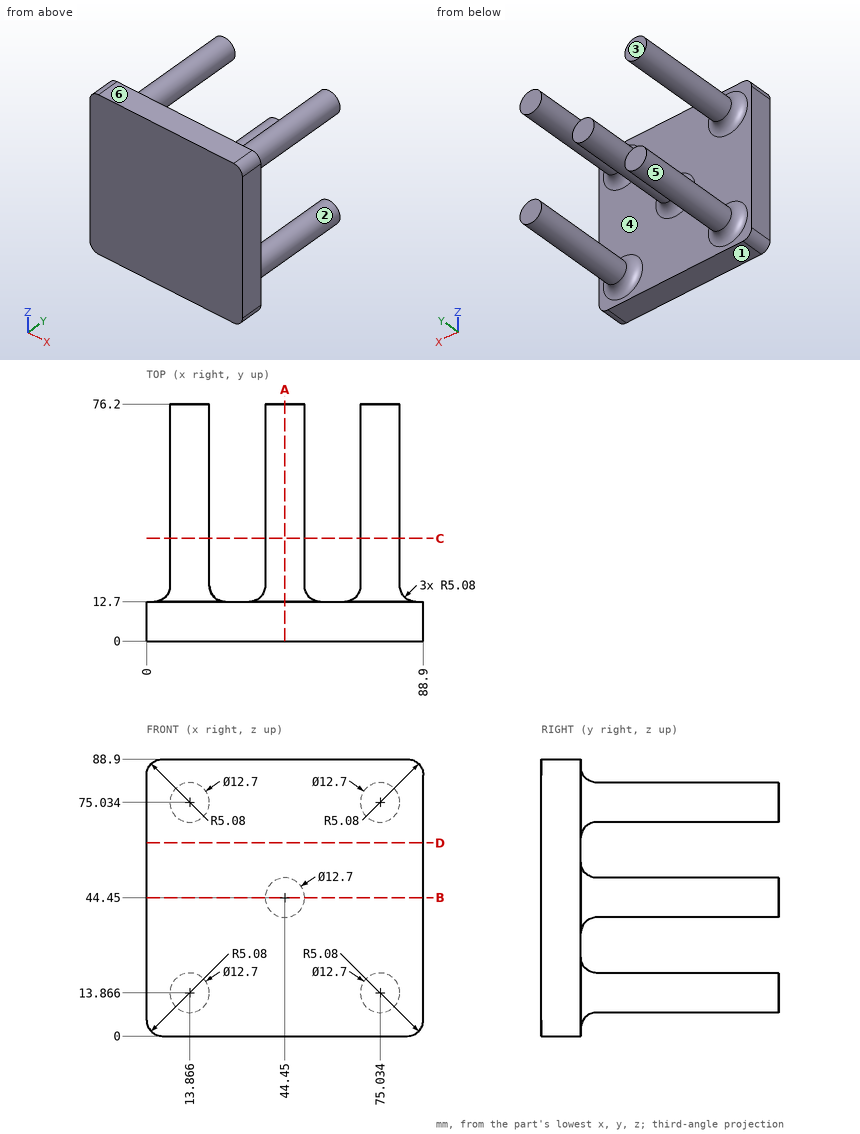
Could you check a few things on this drawing? It's one solid part, dimensions in mm from its lowest x, y, z. A direction names the side the tool comes from. Coordinates: 2 decimals unless noted, no trailing zeros. Order: outer loops, then holes, each group sorted by start corner. A loop starts at its lowest first (then second) coordinate and runs counter-clockwise, first axis right, second up.
1) Imagine slicing it at A-A on x = 44.45. List the corners of the cut face in (y, z) for me, and give its area (3 significant figures).
2) We'd pull the mould along Z, two halves only. Please class the marked faces 1, 2, 3 and 4: +Z half, -Z half, draft (parallel to the pull), parting line (faces both ways), or undercut.
3) Imagine slicing it at B-B on z = 44.45. List the corners of the cut face in (x, y) for me, and give its area (3 significant figures).
4) Imagine slicing it at C-C on y = 33. List the corners of the cut face in (x, z) for me.
5) I need wall thicknesses on line 1 (Y direction, x = 64, z = 65.5); line 2 (X direction, y = 20.5, z = 78.5); line 3 (X direction, y = 25, z = 19.5) (3 decimals). Which ranges of each line are inside material? Lowest first, please.
6) Imagine slicing it at D-D on z = 62. List the corners of the cut face in (x, y) for me.
7) Will these pins go through, and if not, where does the flat tip stop? pin 1 (10 mm diameter, centred on x = 28.5, z = 14, fed in from -Y); pin 2 (2 mm diameter, centred on x = 22.5, z = 43, fed in from +Y); pin 3 (6 mm diameter, centred on x = 52, y = 35.5, fed in from +Z).
8) Which directions (+Z, -Z, +X, -X, +Y, -Y) give clear straight access to the entire face, cutting with the end or side of a thin tool? Please do the marked faces 5 and 6.
Response values:
1. outline: (0, 0) - (12.7, 0) - (12.7, 33.02) arc R5.08 cw to (17.78, 38.1) - (76.2, 38.1) - (76.2, 50.8) - (17.78, 50.8) arc R5.08 cw to (12.7, 55.88) - (12.7, 88.9) - (0, 88.9) - close
1. area: 1,950 mm2
2. face 1: -Z half
2. face 2: undercut
2. face 3: draft
2. face 4: undercut
3. outline: (0, 0) - (88.9, 0) - (88.9, 12.7) - (55.88, 12.7) arc R5.08 cw to (50.8, 17.78) - (50.8, 76.2) - (38.1, 76.2) - (38.1, 17.78) arc R5.08 cw to (33.02, 12.7) - (0, 12.7) - close
3. area: 1,950 mm2
4. outline: circle Ø12.7 at (13.87, 13.87); circle Ø12.7 at (13.87, 75.03); circle Ø12.7 at (44.45, 44.45); circle Ø12.7 at (75.03, 13.87); circle Ø12.7 at (75.03, 75.03)
5. line 1: y = 0 to 12.7
5. line 2: x = 8.55 to 19.19, 69.71 to 80.35
5. line 3: x = 10.937 to 16.795, 72.105 to 77.963
6. outline: (0, 0) - (88.9, 0) - (88.9, 12.7) - (0, 12.7) - close
7. pin 1: stops at y = 0
7. pin 2: stops at y = 12.7
7. pin 3: stops at z = 48.88
8. face 5: +Y
8. face 6: +Z, +X, -X, +Y, -Y
